For this review, take the finished solid that the model builds, in its own axes (mm). Face numbers are marked on the shaded views. A direction names the side the tool comes from. Round coordinates to 2 decimals unless told otherwise and drop trailing zeros. Write each loop counter-clockwise with the first axis right and the second up, starting at its lowest first coordinate (ties: lowest second). Pieces come first, ordered by that corner, then holes. Notation, with made-up numbers: (47, -7) -> (93, -7) arc R28 ccw to (93, 12) -> close; hole circle Ø4 at (48, -13). An arc over 180 degrees is marked (long way). Write each question's results on one line, items separated by ' | '. Start each with the question number.
Item 1: Add section B-B (z = -1.7). State the section outline as (x, y) points (3 decimals), plus the area to 3 significant figures.
Item 2: Clearance check with flat-ended pins moving along their axes: pin 1 (1 mm diameter, centred on y = 1, z = -1.5, fed in from +X); pin 2 (1 mm diameter, centred on y = -0.5, z = -1, fed in from +X); pin 3 (1.3 mm diameter, centred on y = -0.5, z = -1, fed in from -X). State where each tip first meets the part, or that it passes through.
Item 3: Add section A-A (x = 0). State the section outline as (y, z) points (3 decimals).
Item 4: Tool access review of the marked faces 1, 2, 3, 4 and 5: name each direction out of +Z, -Z, +X, -X, +Y, -Y from which nothing blocks a thin tool from reaching the whole face with its end or side.
Item 5: Add section C-C (y = -0.9). State the section outline as (x, z) points, plus the area to 3 significant figures.
Item 6: Add section D-D (x = 1.15). State the section outline as (y, z) points (3 decimals).
Item 7: To check wall thickness, follow line 1 along X through (y, z) = (1.75, 0) (3 decimals); line 2 along Y through (x, z) = (-1, 1.9). State the ranges of each line that lie inside material, in increasing order.
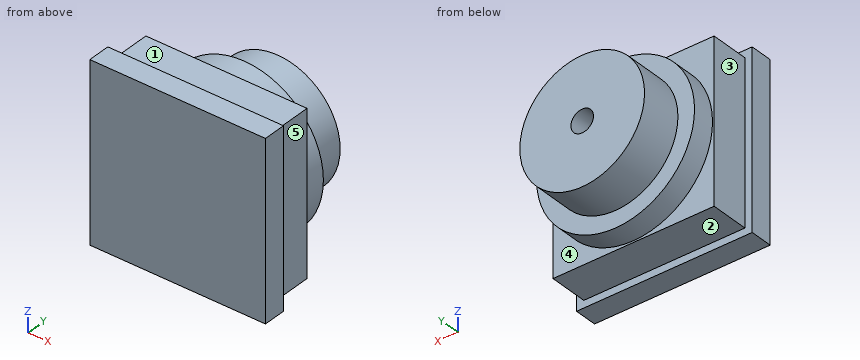
Autodesk Inventor part; units mm, degrees
ref_plane "YZ Plane" through (0, 0, 0) normal (1, 0, 0) x (0, 1, 0)
ref_plane "XZ Plane" through (0, 0, 0) normal (0, 1, 0) x (-1, 0, 0)
ref_plane "XY Plane" through (0, 0, 0) normal (0, 0, 1) x (1, 0, 0)
sketch "Sketch1" plane through (0, 0, 0) normal (0, 1, 0) x (-1, 0, 0)
  circle A0 centre (0, 0) radius 1.935
  dimension "d0" = 3.87
extrude "Extrusion1" add sketch "Sketch1" along normal blind 2
sketch "Sketch2" plane through (0, 0, 0) normal (0, -1, 0) x (1, 0, 0)
  line L0 (2.5, 2.5) -> (-2.5, 2.5)
  line L1 (-2.5, 2.5) -> (-2.5, -2.5)
  line L2 (-2.5, -2.5) -> (2.5, -2.5)
  line L3 (2.5, -2.5) -> (2.5, 2.5)
  line L4 (2.5, 2.5) -> (-2.5, -2.5) construction
  line L5 (-2.5, 2.5) -> (2.5, -2.5) construction
  point P0 (0, 0)
  dimension "d9" = 5
  dimension "d10" = 5
extrude "Extrusion2" add sketch "Sketch2" along normal blind 1.2
sketch "Sketch3" plane through (0, -1.2, 0) normal (0, -1, 0) x (1, 0, 0)
  line L0 (2.725, 2.725) -> (-2.725, 2.725)
  line L1 (-2.725, 2.725) -> (-2.725, -2.725)
  line L2 (-2.725, -2.725) -> (2.725, -2.725)
  line L3 (2.725, -2.725) -> (2.725, 2.725)
  line L4 (2.725, 2.725) -> (-2.725, -2.725) construction
  line L5 (-2.725, 2.725) -> (2.725, -2.725) construction
  point P0 (0, 0)
  dimension "d5" = 5.45
  dimension "d6" = 5.45
extrude "Extrusion3" add sketch "Sketch3" along normal blind 0.7
sketch "Sketch4" plane through (0, 0, 0) normal (0, 1, 0) x (1, 0, 0)
  circle A0 centre (0, 0) radius 2.45
  dimension "d11" = 4.9
extrude "Extrusion4" add sketch "Sketch4" along normal blind 0.7
sketch "Sketch5" plane through (0, 2, 0) normal (0, 1, 0) x (1, 0, 0)
  circle A0 centre (0, 0) radius 0.35
  dimension "d14" = 0.7
extrude "Extrusion5" cut sketch "Sketch5" against normal blind 0.7
properties part number "Camera"
Responses:
1) outline: (-2.725, -1.9) -> (2.725, -1.9) -> (2.725, -1.2) -> (2.5, -1.2) -> (2.5, 0) -> (1.764, 0) -> (1.764, 0.7) -> (0.924, 0.7) -> (0.924, 2) -> (-0.924, 2) -> (-0.924, 0.7) -> (-1.764, 0.7) -> (-1.764, 0) -> (-2.5, 0) -> (-2.5, -1.2) -> (-2.725, -1.2) -> close | area: 14.7 mm^2
2) pin 1: stops at x = 2.19 | pin 2: stops at x = 2.5 | pin 3: stops at x = -2.5
3) outline: (-1.9, -2.725) -> (-1.2, -2.725) -> (-1.2, -2.5) -> (0, -2.5) -> (0, -2.45) -> (0.7, -2.45) -> (0.7, -1.935) -> (2, -1.935) -> (2, -0.35) -> (1.3, -0.35) -> (1.3, 0.35) -> (2, 0.35) -> (2, 1.935) -> (0.7, 1.935) -> (0.7, 2.45) -> (0, 2.45) -> (0, 2.5) -> (-1.2, 2.5) -> (-1.2, 2.725) -> (-1.9, 2.725) -> close
4) face 1: +Z, +X, -X, +Y | face 2: -Z, +X, -X, +Y | face 3: +Z, -Z, -X, +Y | face 4: +Y | face 5: +Z, -Z, +X, +Y
5) outline: (-2.5, -2.5) -> (2.5, -2.5) -> (2.5, 2.5) -> (-2.5, 2.5) -> close | area: 25.0 mm^2
6) outline: (-1.9, -2.725) -> (-1.2, -2.725) -> (-1.2, -2.5) -> (0, -2.5) -> (0, -2.163) -> (0.7, -2.163) -> (0.7, -1.556) -> (2, -1.556) -> (2, 1.556) -> (0.7, 1.556) -> (0.7, 2.163) -> (0, 2.163) -> (0, 2.5) -> (-1.2, 2.5) -> (-1.2, 2.725) -> (-1.9, 2.725) -> close
7) line 1: x = -1.935 to -0.35, 0.35 to 1.935 | line 2: y = -1.9 to 0.7
